Can you work these out from the model? Positions are in its coordinate system, mm. A direction names the side the tool comes from. Give positions to 0.01 mm unless a question says otherwise; leave off trailing zeros. Loops run counter-clockwise (first coordinate to the right, second up) from the corner with the lowest first, then second, coordinate; pieces in that order, holes last. Notation, with made-up numbers: (14.5, -1) - (53.5, -1) arc R36 ccw to (53.5, 38) - close; hole circle Ø10 at (73.5, 86.25). An arc over 180 degrees is marked (long way). Answer as a JSON object with one key per item and string values.
```python
from build123d import *

# Parameters (mm, degrees)
SKETCH_1_W          = 7
SKETCH_1_H          = 9
EXTRUDE_1_DEPTH     = 10
SKETCH_2_R          = 2.2
CUT_EXTRUDE_1_DEPTH = 10
EXTRUDE_2_DEPTH     = 7
CUT_EXTRUDE_2_DEPTH = 7
FILLET_2_R          = 1.5
FILLET_3_R          = 1.5
FILLET_4_R          = 1.5


with BuildPart() as part:
    # 草图1 → 凸台-拉伸1 (new body)
    with BuildSketch(Plane(origin=(0, 0, 0), x_dir=(1, 0, 0), z_dir=(0, 1, 0))):
        Rectangle(SKETCH_1_W, SKETCH_1_H)
    extrude(amount=EXTRUDE_1_DEPTH)

    # 草图2 → 切除-拉伸1 (cut)
    with BuildSketch(Plane(origin=(0, 10, 0), x_dir=(1, 0, 0), z_dir=(0, 1, 0))):
        Circle(SKETCH_2_R)
    extrude(amount=-CUT_EXTRUDE_1_DEPTH, mode=Mode.SUBTRACT)

    # 草图3 → 凸台-拉伸2 (add)
    with BuildSketch(Plane.ZY.offset(3.5)):
        Polygon((4.5, 10), (4.5, 0), (62.235026919, -100), (77.235026919, -100), (77.235026919, -95), (65.121778265, -95), align=None)
    extrude(amount=-EXTRUDE_2_DEPTH)

    # 草图4 → 切除-拉伸2 (cut)
    with BuildSketch(Plane.ZY.offset(3.5)):
        Polygon((4.5, 0), (1.613248654, 5), (-4.5, 5), (-4.5, 0), align=None)
    extrude(amount=-CUT_EXTRUDE_2_DEPTH, mode=Mode.SUBTRACT)

    # 圆角2
    fillet_2_edges = [part.edges().sort_by_distance(p)[0] for p in [
        (0, 10, 4.5),
    ]]
    fillet(fillet_2_edges, radius=FILLET_2_R)

    # 圆角3
    fillet_3_edges = [part.edges().sort_by_distance(p)[0] for p in [
        (2.497901862, 5, 1.613248654),
        (-2.497901862, 5, 1.613248654),
    ]]
    fillet(fillet_3_edges, radius=FILLET_3_R)

    # 圆角4
    fillet_4_edges = [part.edges().sort_by_distance(p)[0] for p in [
        (0, -100, 77.235026919),
        (0, -100, 62.235026919),
        (0, -95, 65.121778265),
        (0, -95, 77.235026919),
    ]]
    fillet(fillet_4_edges, radius=FILLET_4_R)


solid = part.part
```
1) Which directions (+Z, -Z, +X, -X, +Y, -Y) give clear straight access to the entire face, cutting with the end or side of a thin tool? Please do faces 1 (the flat face through (0.7, 10, -2.3)), 2 (the flat face through (0, -95, 71)).
Check sheet entries:
{"face 1": "+Z, -Z, +X, -X, +Y", "face 2": "+Z, +X, -X, +Y"}
2) Imagine slicing it at A-A on y = -39. Write out the boundary of the cut face in (x, z).
Check sheet entries:
{"outline": "(-3.5, 27.02) - (3.5, 27.02) - (3.5, 32.79) - (-3.5, 32.79) - close"}
3) If we mould it in two halves opening along Z, with no side actions, what happens to faces 3 (the flat face through (-0.049, -43.224, 35.229)), 4 (the flat face through (0, 7, -4.5)), 5 (the cylindrical face through (-0.477, 7.688, 2.148)), 6 (the flat face through (0, 5, -2.4))? For each: released by +Z, released by -Z, zero draft, split by the parting line, or undercut.
Check sheet entries:
{"face 3": "released by +Z", "face 4": "released by -Z", "face 5": "undercut", "face 6": "zero draft"}
4) Imagine slicing it at B-B on z = 30. Write out the boundary of the cut face in (x, y).
Check sheet entries:
{"outline": "(-3.5, -44.17) - (3.5, -44.17) - (3.5, -34.17) - (-3.5, -34.17) - close"}
5) I'm going to push flat-ended pins straight in: P1, Ø2, axis at x = 1.5, z = 72, coming from the +Y side; P2, Ø4, axis at x = 1.5, y = -3, coming from the -Z side; P3, Ø4, axis at x = -1.5, z = -2, coming from the -Y side. Where does each tip first touch, or does it pass through?
Check sheet entries:
{"P1": "y = -95", "P2": "z = 5.08", "P3": "y = 5"}
6) I need wall thicknesses on L1, parallel to X at y = 6.25, z = 0; L2, parallel to Y at x = 0.75, z = 69; L3, parallel to Z at x = 0, y = 8.75. Which ranges of each line are inside material? Lowest first, please.
Check sheet entries:
{"L1": "-3.5 to -2.2, 2.2 to 3.5", "L2": "-100 to -95", "L3": "-4.5 to -2.2, 2.2 to 5.22"}
